Verification items for the finished model (mm, model axes). Face numbers are marked on the shaded views. A direction names the side the tool comes from. Coordinates: 2 decimals unless noted, no trailing zeros. Order: outer loops, then holes, each group sorted by start corner. A loop starts at its lowest first (then second) coordinate and runs counter-clockwise, first axis right, second up. Notation, with made-up numbers: (-5, -34.5) -> (53, -34.5) arc R29 cw to (53, 2.5) -> close; hole circle Ø8 at (84, 72.5). An arc over 180 degrees is marked (long way). Answer as CSV lines item,"result".
```python
from build123d import *

# Parameters (mm, degrees)
BOSS_EXTRUDE2_DEPTH            = 40
M5_CLEARANCE_HOLE2_D           = 5.5
M5_CLEARANCE_HOLE2_CSINK_D     = 5.55
M5_CLEARANCE_HOLE2_CSINK_ANGLE = 90
CUT_EXTRUDE1_REACH             = 277.363
SKETCH10_R                     = 16
CUT_EXTRUDE2_DEPTH             = 10
CUT_EXTRUDE2_DEPTH_BACK        = 9
SKETCH12_R                     = 18.6
FILLET1_START                  = -1
FILLET1_DEPTH                  = 192.875384615
FILLET1_START_2                = -186
FILLET1_2_DEPTH                = 178.689653846
M5_CLEARANCE_HOLE3_D           = 5.5
M5_CLEARANCE_HOLE3_CSINK_D     = 5.55
M5_CLEARANCE_HOLE3_CSINK_ANGLE = 90


with BuildPart() as part:
    # Sketch6 → Boss-Extrude2 (new body)
    with BuildSketch(Plane(origin=(0, 0, 0), x_dir=(0, 0, -1), z_dir=(1, 0, 0))):
        with BuildLine():
            Line((0, 0), (40, 0))
            ThreePointArc((40, 0), (142.530483272, 42.469516728), (185, 145))
            Line((185, 145), (185, 200))
            Line((185, 200), (170, 200))
            Line((170, 200), (170, 145))
            ThreePointArc((170, 145), (131.923881554, 53.076118446), (40, 15))
            Line((40, 15), (0, 15))
            Line((0, 15), (0, 0))
        make_face()
    extrude(amount=BOSS_EXTRUDE2_DEPTH)

    # M5 Clearance Hole2 (through all)
    with Locations(Plane(origin=(0, 15, 0), x_dir=(1, 0, 0), z_dir=(0, 1, 0))):
        with Locations((10, 30), (30, 30), (10, 10), (30, 10)):
            CounterSinkHole(M5_CLEARANCE_HOLE2_D / 2, M5_CLEARANCE_HOLE2_CSINK_D / 2, counter_sink_angle=M5_CLEARANCE_HOLE2_CSINK_ANGLE)

    # Sketch10 → Cut-Extrude1 (cut, up to next)
    with BuildSketch(Plane(origin=(0, 0, -185), x_dir=(-1, 0, 0), z_dir=(0, 0, -1)), mode=Mode.PRIVATE) as cut_extrude1_sk1:
        with Locations(Location((-20, 160, 0), (0, 0, 290.364134806))):
            Circle(SKETCH10_R)
    cut_extrude1_tool1 = extrude(cut_extrude1_sk1.sketch, amount=-CUT_EXTRUDE1_REACH, mode=Mode.PRIVATE) & part.part
    add(cut_extrude1_tool1.solids().sort_by_distance((20, 160, -185))[0], mode=Mode.SUBTRACT)

    # Sketch12 → Cut-Extrude2 (cut, two sides: drawn at the far end of the back side and taken through both)
    with BuildSketch(Plane.XY.offset(-170).offset(-CUT_EXTRUDE2_DEPTH_BACK)):
        with Locations(Location((20, 160, 0), (0, 0, 233.750679117))):
            Circle(SKETCH12_R)
    extrude(amount=CUT_EXTRUDE2_DEPTH + CUT_EXTRUDE2_DEPTH_BACK, mode=Mode.SUBTRACT)

    # Fillet1: read off the stored shape, not the designer's step
    # Fillet1 outline → Fillet1 (cut)
    with BuildSketch(Plane(origin=(0, 0, 0), x_dir=(1, 0, 0), z_dir=(0, 1, 0)).offset(FILLET1_START)):
        with BuildLine():
            Line((40, 0), (40, 10))
            add(Edge.make_bspline(
                [(40, 10), (40, 0), (30, 0)],
                knots=[0, 0, 0, 1, 1, 1], degree=2, weights=[1, 0.707106781, 1]))
            Line((30, 0), (40, 0))
        make_face()
        with BuildLine():
            Line((0, 0), (10, 0))
            add(Edge.make_bspline(
                [(10, 0), (0, 0), (0, 10)],
                knots=[0, 0, 0, 1, 1, 1], degree=2, weights=[1, 0.707106781, 1]))
            Line((0, 10), (0, 0))
        make_face()
    extrude(amount=FILLET1_DEPTH, mode=Mode.SUBTRACT)

    # Fillet1 2 outline → Fillet1 2 (cut)
    with BuildSketch(Plane.XY.offset(FILLET1_START_2)):
        with BuildLine():
            add(Edge.make_bspline(
                [(10, 200), (0, 200), (0, 190)],
                knots=[0, 0, 0, 1, 1, 1], degree=2, weights=[1, 0.707106781, 1]))
            Line((10, 200), (0, 200))
            Line((0, 200), (0, 190))
        make_face()
        with BuildLine():
            add(Edge.make_bspline(
                [(40, 190), (40, 200), (30, 200)],
                knots=[0, 0, 0, 1, 1, 1], degree=2, weights=[1, 0.707106781, 1]))
            Line((40, 190), (40, 200))
            Line((40, 200), (30, 200))
        make_face()
    extrude(amount=FILLET1_2_DEPTH, mode=Mode.SUBTRACT)

    # M5 Clearance Hole3 (through all)
    with Locations(Plane(origin=(0, 0, -185), x_dir=(-1, 0, 0), z_dir=(0, 0, -1))):
        with Locations((-30, 190), (-10, 190)):
            CounterSinkHole(M5_CLEARANCE_HOLE3_D / 2, M5_CLEARANCE_HOLE3_CSINK_D / 2, counter_sink_angle=M5_CLEARANCE_HOLE3_CSINK_ANGLE)


solid = part.part
```
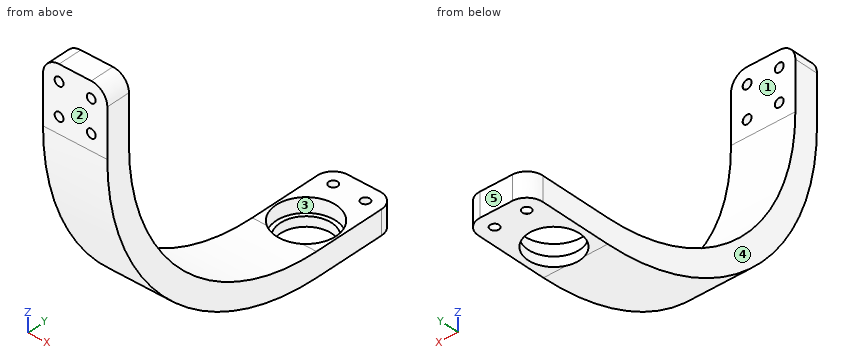
Item 1: Thickness scan on line 1 (X direction, y = 6.5, z = -30); line 2 (Z direction, x = 10, y = 11); line 3 (X direction, y = 160, z = -176). Record the ranges inside material, lowest first.
Answer list:
line 1,"0 to 7.25, 12.75 to 27.25, 32.75 to 40"
line 2,"-95.4 to -32.75, -27.25 to -12.75, -7.25 to 0"
line 3,"0 to 1.4, 38.6 to 40"
Item 2: Tool access check on the marked faces 1 and 2. Record the directions out of +Z, -Z, +X, -X, +Y, -Y that give a thin tool (end or side, any length) a straight path to the whole face; none if there is none.
Answer list:
face 1,"+Z, +X, -X, +Y"
face 2,"+Z, -Z, +X, -X, -Y"
Item 3: Section check B-B, the plane x = 18. Record the boundary of the cut face in (y, z), plus the area to 3 significant figures.
Answer list:
outline,"(0, -40) arc R145 ccw to (144.13, -185) -> (144.13, -179) -> (141.51, -179) -> (141.51, -169.95) arc R130 cw to (15, -40) -> (15, 0) -> (0, 0) -> close; (175.87, -185) -> (200, -185) -> (200, -170) -> (178.49, -170) -> (178.49, -179) -> (175.87, -179) -> close"
area,"4,140 mm2"
Item 4: Section check C-C, the plane y = 116.5. Record the boundary of the cut face in (x, z).
Answer list:
outline,"(0, -182.17) -> (40, -182.17) -> (40, -166.84) -> (0, -166.84) -> close"
Item 5: Section check A-A, the plane z = -30. Record the boundary of the cut face in (x, y) (3 decimals), plus the area to 3 significant figures.
Answer list:
outline,"(0, 0) -> (7.25, 0) -> (7.25, 14.975) -> (7.225, 15) -> (0, 15) -> close; (12.75, 0) -> (27.25, 0) -> (27.25, 14.975) -> (27.225, 15) -> (12.775, 15) -> (12.75, 14.975) -> close; (32.75, 0) -> (40, 0) -> (40, 15) -> (32.775, 15) -> (32.75, 14.975) -> close"
area,"435 mm2"
Item 6: Release check for a two-part mould opening along X. For the marked faces 3, 4 and 5 record: +X half, -X half, draft (parallel to the pull), parting line (faces both ways), or undercut.
Answer list:
face 3,"undercut"
face 4,"-X half"
face 5,"draft"
Item 7: Section check D-D, the plane z = -156. Record the boundary of the cut face in (x, y).
Answer list:
outline,"(0, 58) -> (40, 58) -> (40, 86.31) -> (0, 86.31) -> close"
Item 8: Depth check by flat-ended pin: pin 1 Ø12 at (y, z) = (21, -125) entering from +X; pin 2 Ø3.5 at (x, y) = (10, 190) entering from -Z; pin 3 Ø5 at (x, y) = (11, 86) entering from +Z; pin 4 Ø7 at (x, y) = (30, 190) entering from +Z. Enter the tip coordinate at first touch or a pass-through.
Answer list:
pin 1,"x = 40"
pin 2,"through"
pin 3,"z = -154.53"
pin 4,"z = -170"
